For this review, take the finished solid that the model builds, in its own axes (mm). A direction names the side the tool comes from. Coordinates: 2 decimals unless noted, no trailing zeros. Write each loop counter-clockwise with the first axis right and the second up, starting at its lowest first coordinate (ties: lowest second). Pieces come first, ordered by that corner, then holes. Notation, with made-up numbers: (6, 40.25) - (13, 40.25) arc R23 ccw to (13, 73.25) - close; hole circle Ø3 at (29, -7). An arc over 180 degrees is marked (long way). Use one line per item in the form item = value. Start each with the question number.
1) We need section C-C (y = 0). Give the boundary of the cut face in (x, z).
2) We need section D-D (x = -24). Give the boundary of the cut face in (y, z), plus the area to 3 significant figures.
3) Mouldability with a two-part tool opening along X and no side actions: class faces 1 (the flat face through (-4.29, 11.36, 1.66)), 2 (the cylindrical face through (-20.734, 21.842, 2.465)), 3 (the flat face through (0, 22, 5)), 4 (the cylindrical face through (27.985, 24.744, 2.465)) as pulls with the +X half, pulls with the -X half, needs draft (parallel to the pull), parting line crosses it, or undercut.
4) Insertion check: P1, Ø2.5, axis at x = -1.5, z = 2.5, coming from the -Y side; P2, Ø4.5, axis at x = -22.63, y = 22.63, coming from the -Z side; P3, Ø5, axis at x = -7, y = 10, coming from the +Z side; P4, Ø1, axis at x = 6.5, z = 4, coming from the -Y side. Each pin has a flat end and moves straight along its axis. Give the tip position at first contact, or say it passes through.
5) We need section B-B (z = 0.75). Give the boundary of the cut face in (x, y), plus the area to 3 significant figures.
6) We need section A-A (x = 0). Give the boundary of the cut face in (y, z).
7) Tool access review of faces 5 (the flat face through (0, 28.388, 2)), 6 (the flat face through (-8.09, 17.28, 4.19)), 7 (the cylindrical face through (-7.49, 16.39, 1.91)): name each direction out of +Z, -Z, +X, -X, +Y, -Y from which nothing blocks a thin tool from reaching the whole face with its end or side.
8) For L1, parallel to Y at x = 0, z = 0.8; L2, parallel to X at y = 24.5, z = 2.95; L3, parallel to X at y = 13, z = 1.9, list the stretches that pass through material, from the lowest coordinate up. Write a range as from..to.
```python
from build123d import *

# Parameters (mm, degrees)
SCHIZZO1_R                   = 2.05
ESTRUSIONE_ESTRUSIONE1_DEPTH = 5
CUT_EXTRUDE2_DEPTH           = 1.64


with BuildPart() as part:
    # Schizzo1 → Estrusione-Estrusione1 (new body)
    with BuildSketch(Plane.XY):
        with BuildLine():
            Line((22.627416998, 28.387976608), (-22.627416998, 28.387976608))
            ThreePointArc((-22.627416998, 28.387976608), (-27.949480117, 24.831887722), (-26.700747761, 18.554086235))
            Line((-26.700747761, 18.554086235), (-4.073330763, -4.073330763))
            ThreePointArc((-4.073330763, -4.073330763), (0, -5.76055961), (4.073330763, -4.073330763))
            Line((4.073330763, -4.073330763), (26.700747761, 18.554086235))
            ThreePointArc((26.700747761, 18.554086235), (27.949480117, 24.831887722), (22.627416998, 28.387976608))
        make_face()
        Circle(SCHIZZO1_R, mode=Mode.SUBTRACT)
        with Locations((22.627416998, 22.627416998)):
            Circle(SCHIZZO1_R, mode=Mode.SUBTRACT)
        with Locations((-22.627416998, 22.627416998)):
            Circle(SCHIZZO1_R, mode=Mode.SUBTRACT)
        with BuildLine():
            Line((5.607211383, 17.627416998), (-5.607211383, 17.627416998))
            ThreePointArc((-5.607211383, 17.627416998), (-7.501164425, 16.361918034), (-7.056780285, 14.127848097))
            Line((-7.056780285, 14.127848097), (-1.449568901, 8.520636713))
            ThreePointArc((-1.449568901, 8.520636713), (0, 7.920205615), (1.449568901, 8.520636713))
            Line((1.449568901, 8.520636713), (7.056780285, 14.127848097))
            ThreePointArc((7.056780285, 14.127848097), (7.501164425, 16.361918034), (5.607211383, 17.627416998))
        make_face(mode=Mode.SUBTRACT)
    extrude(amount=ESTRUSIONE_ESTRUSIONE1_DEPTH)

    # Sketch2 → Cut-Extrude2 (cut)
    with BuildSketch(Plane.XY.offset(5)):
        Polygon((12.797266468, 4.650604941), (0, -8.146661527), (-19.643815137, 11.49715361), (-9.946322881, 17.017390693), (-5.607211383, 17.627416998), (-1.449568901, 8.520636713), (1.449568901, 8.520636713), (5.188401798, 12.25946961), align=None)
    extrude(amount=-CUT_EXTRUDE2_DEPTH, mode=Mode.SUBTRACT)


solid = part.part
```
Determined:
q1.outline = (-8.15, 0) - (-2.05, 0) - (-2.05, 3.36) - (-8.15, 3.36) - close; (2.05, 0) - (8.15, 0) - (8.15, 3.36) - (2.05, 3.36) - close
q2.outline = (15.85, 0) - (21.1, 0) - (21.1, 5) - (15.85, 5) - close; (24.15, 0) - (28.22, 0) - (28.22, 5) - (24.15, 5) - close
q2.area = 46.6 mm²
q3.face_1 = undercut
q3.face_2 = undercut
q3.face_3 = needs draft
q3.face_4 = pulls with the +X half
q4.P1 = -5.76
q4.P2 = 0
q4.P3 = 3.36
q4.P4 = 10.45
q5.outline = (-26.7, 18.55) - (-4.07, -4.07) arc R5.76 ccw to (4.07, -4.07) - (26.7, 18.55) arc R5.76 ccw to (22.63, 28.39) - (-22.63, 28.39) arc R5.76 ccw to start; hole circle Ø4.1 at (-22.63, 22.63); hole (-7.06, 14.13) - (-1.45, 8.52) arc R2.05 ccw to (1.45, 8.52) - (7.06, 14.13) arc R2.05 ccw to (5.61, 17.63) - (-5.61, 17.63) arc R2.05 ccw to start; hole circle Ø4.1 at (0, 0); hole circle Ø4.1 at (22.63, 22.63)
q5.area = 1,110 mm²
q6.outline = (-5.76, 0) - (-2.05, 0) - (-2.05, 3.36) - (-5.76, 3.36) - close; (2.05, 0) - (7.92, 0) - (7.92, 3.36) - (2.05, 3.36) - close; (17.63, 0) - (28.39, 0) - (28.39, 5) - (17.63, 5) - close
q7.face_5 = +Z, -Z, +X, -X, +Y
q7.face_6 = +Z, -Y
q7.face_7 = +Z, -Z
q8.L1 = -5.76..-2.05, 2.05..7.92, 17.63..28.39
q8.L2 = -28.08..-23.46, -21.79..21.79, 23.46..28.08
q8.L3 = -21.15..-5.93, 5.93..21.15
